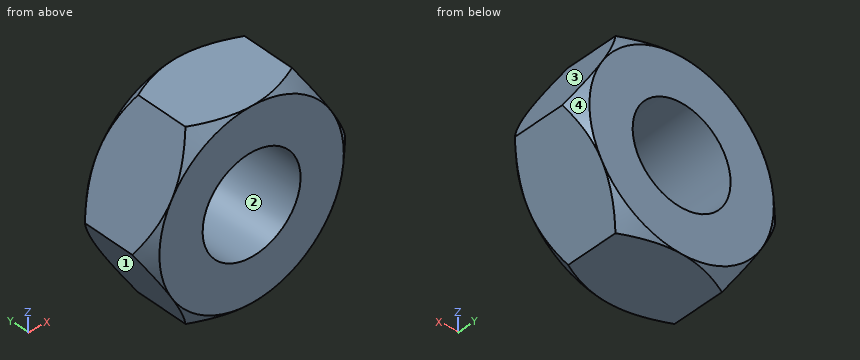
from build123d import *

# Parameters (mm, degrees)
EXTRUDE1_DEPTH                   = 5.6
SKETCH3_R                        = 12.424094019
SKETCH3_R_2                      = 6.4
EXTRUDE3_DEPTH                   = 6.1
EXTRUDE3_TAPER                   = 45
SKETCH4_R                        = 12.424094019
SKETCH4_R_2                      = 6.4
EXTRUDE4_DEPTH                   = 6.1
EXTRUDE4_DRAFT                   = -45
TAP_DRILL_FOR_M8X1_25_TAP1_D     = 6.8
TAP_DRILL_FOR_M8X1_25_TAP1_DEPTH = 10
TAP_DRILL_FOR_M8X1_25_TAP1_TIP   = 2.042926105


with BuildPart() as part:
    # Sketch1 → Extrude1 (new body)
    with BuildSketch(Plane(origin=(0, 0, 0), x_dir=(1, 0, 0), z_dir=(0, 1, 0))):
        Polygon((7.390083446, 0), (3.695041723, 6.4), (-3.695041723, 6.4), (-7.390083446, 0), (-3.695041723, -6.4), (3.695041723, -6.4), align=None)
    extrude(amount=EXTRUDE1_DEPTH)

    # Sketch3 → Extrude3 (cut)
    with BuildSketch(Plane(origin=(0, 5.6, 0), x_dir=(1, 0, 0), z_dir=(0, 1, 0))):
        Circle(SKETCH3_R)
        Circle(SKETCH3_R_2, mode=Mode.SUBTRACT)
    extrude(amount=-EXTRUDE3_DEPTH, taper=EXTRUDE3_TAPER, mode=Mode.SUBTRACT)


with BuildPart() as extrude4_tool:
    # Sketch4 → Extrude4 (with draft: the straight prism first)
    with BuildSketch(Plane.XZ):
        Circle(SKETCH4_R)
        Circle(SKETCH4_R_2, mode=Mode.SUBTRACT)
    extrude(amount=-EXTRUDE4_DEPTH)
    # Extrude4: the draft: its side faces are tilted about the plane it starts from
    extrude4_sides = [extrude4_tool.faces().sort_by_distance(p)[0] for p in [
        (-12.424094019, 3.05, 0),
        (-6.4, 3.05, 0),
    ]]
    draft(extrude4_sides, Plane.XZ, EXTRUDE4_DRAFT)


with BuildPart() as part_1:
    add(part.part)

    # Extrude4: cut by extrude4_tool
    add(extrude4_tool.part, mode=Mode.SUBTRACT)

    # Tap Drill for M8x1.25 Tap1
    with Locations(Plane.ZX.offset(5.6)):
        with Locations((0, 0)):
            Hole(TAP_DRILL_FOR_M8X1_25_TAP1_D / 2, depth=TAP_DRILL_FOR_M8X1_25_TAP1_DEPTH)
            with Locations((0, 0, -(TAP_DRILL_FOR_M8X1_25_TAP1_DEPTH + TAP_DRILL_FOR_M8X1_25_TAP1_TIP / 2))):  # 118° drill point
                Cone(0, TAP_DRILL_FOR_M8X1_25_TAP1_D / 2, TAP_DRILL_FOR_M8X1_25_TAP1_TIP, mode=Mode.SUBTRACT)


solid = part_1.part
Verification items for the finished model (mm, model axes). Face numbers are marked on the shaded views. Coordinates: 2 decimals unless noted, no trailing zeros. Loops run counter-clockwise (first coordinate to the right, second up) from the corner with the lowest first, then second, coordinate; pieces in that order, holes last. Notation, with made-up numbers: M 78.5,21 L 89.5,21 A27 ccw 89.5,57 Z; hole C 38.25,53.5 d3. An arc over 180 degrees is marked long. One line per item, written item: value.
1. Mould release check, pull along Z, two halves, no side actions. Record for the marked faces 1, 2, 3 and 4: pulls with the +Z half, pulls with the -Z half, needs draft (parallel to the pull), parting line crosses it, or undercut.
Answers follow:
face 1: pulls with the -Z half
face 2: undercut
face 3: pulls with the +Z half
face 4: parting line crosses it
2. Gauge pin test, flat end, axial feed: P1, Ø1, axis at y = 3, z = -2.5, coming from the -X side. Record the tip position at first contact, or that the pin passes through.
Answers follow:
P1: x = -6.24
3. Material ranges on line 1 along X through (y, z) = (4.9, -2.75); line 2 along Z through (x, y) = (-2, 3.7); line 3 along Z through (x, y) = (2.5, 2.2), recorded low to high. Write a range as from..to.
Answers follow:
line 1: -5.8..-2, 2..5.8
line 2: -6.4..-2.75, 2.75..6.4
line 3: -6.4..-2.3, 2.3..6.4
4. Section check A-A on y = 3.9. Record the cut outline in (x, z), plus the area to 3 significant figures.
Answers follow:
outline: M -7.39,0 L -3.7,-6.4 L 3.7,-6.4 L 7.39,0 L 3.7,6.4 L -3.7,6.4 Z; hole C 0,0 d6.8
area: 106 mm^2
